from build123d import *

# Parameters (mm, degrees)
BASE_FLANGE1_DEPTH      = 4.4
CUT_EXTRUDE1_DEPTH      = 10.36
CUT_EXTRUDE1_DEPTH_BACK = 4.76
CUT_EXTRUDE2_DEPTH      = 4.76
BOSS_EXTRUDE1_START     = 0.36
BOSS_EXTRUDE1_DEPTH     = 0.36


# Sheet-metal steps are written as plain solids
with BuildPart() as part:
    # Sketch2 → Base-Flange1 (new body)
    with BuildSketch(Plane(origin=(0, 0, 0), x_dir=(1, 0, 0), z_dir=(0, 1, 0))):
        with BuildLine():
            Line((-33.306696524, 16.994496658), (30.293303476, 16.994496658))
            ThreePointArc((30.293303476, 16.994496658), (32.556045176, 16.057238357), (33.493303476, 13.794496658))
            Line((33.493303476, 13.794496658), (33.493303476, -9.805503342))
            ThreePointArc((33.493303476, -9.805503342), (32.556045176, -12.068245042), (30.293303476, -13.005503342))
            Line((30.293303476, -13.005503342), (-33.306696524, -13.005503342))
            ThreePointArc((-33.306696524, -13.005503342), (-35.569438223, -12.068245042), (-36.506696524, -9.805503342))
            Line((-36.506696524, -9.805503342), (-36.506696524, 13.794496658))
            ThreePointArc((-36.506696524, 13.794496658), (-35.569438223, 16.057238357), (-33.306696524, 16.994496658))
        make_face()
    extrude(amount=-BASE_FLANGE1_DEPTH)

    # Sketch7 → Cut-Extrude1 (cut, two sides: drawn at the far end of the back side and taken through both)
    with BuildSketch(Plane(origin=(0, 0, 0), x_dir=(1, 0, 0), z_dir=(0, 1, 0)).offset(-CUT_EXTRUDE1_DEPTH_BACK)):
        with BuildLine():
            Line((-28.006696524, 4.494496658), (-19.506696524, 4.494496658))
            ThreePointArc((-19.506696524, 4.494496658), (-17.006696524, 1.994496658), (-19.506696524, -0.505503342))
            Line((-19.506696524, -0.505503342), (-28.006696524, -0.505503342))
            ThreePointArc((-28.006696524, -0.505503342), (-30.506696524, 1.994496658), (-28.006696524, 4.494496658))
        make_face()
        with BuildLine():
            Line((23.493303476, 4.494496658), (33.493303476, 4.494496658))
            ThreePointArc((33.493303476, 4.494496658), (35.993303476, 1.994496658), (33.493303476, -0.505503342))
            Line((33.493303476, -0.505503342), (23.493303476, -0.505503342))
            ThreePointArc((23.493303476, -0.505503342), (20.993303476, 1.994496658), (23.493303476, 4.494496658))
        make_face()
    extrude(amount=CUT_EXTRUDE1_DEPTH + CUT_EXTRUDE1_DEPTH_BACK, mode=Mode.SUBTRACT)

    # Sketch8 → Cut-Extrude2 (cut)
    with BuildSketch(Plane(origin=(0, 0, 0), x_dir=(1, 0, 0), z_dir=(0, 1, 0))):
        with BuildLine():
            Line((8.293303476, 2.994496658), (8.293303476, -13.005503342))
            ThreePointArc((8.293303476, -13.005503342), (1.993303476, -19.305503342), (-4.306696524, -13.005503342))
            Line((-4.306696524, -13.005503342), (-4.306696524, 2.994496658))
            ThreePointArc((-4.306696524, 2.994496658), (1.993303476, 9.294496658), (8.293303476, 2.994496658))
        make_face()
    extrude(amount=-CUT_EXTRUDE2_DEPTH, mode=Mode.SUBTRACT)

    # Sketch11 → Boss-Extrude1 (add)
    with BuildSketch(Plane(origin=(0, 0, 0), x_dir=(1, 0, 0), z_dir=(0, 1, 0)).offset(BOSS_EXTRUDE1_START)):
        with BuildLine():
            Line((-36.506696524, 13.794496658), (-36.506696524, -9.805503342))
            ThreePointArc((-36.506696524, -9.805503342), (-35.569438223, -12.068245042), (-33.306696524, -13.005503342))
            Line((-33.306696524, -13.005503342), (-7.006696524, -13.005503342))
            Line((-7.006696524, -13.005503342), (-7.006696524, 2.994496658))
            ThreePointArc((-7.006696524, 2.994496658), (1.993303476, 11.994496658), (10.993303476, 2.994496658))
            Line((10.993303476, 2.994496658), (10.993303476, -13.005503342))
            Line((10.993303476, -13.005503342), (30.293303476, -13.005503342))
            ThreePointArc((30.293303476, -13.005503342), (32.556045176, -12.068245042), (33.493303476, -9.805503342))
            Line((33.493303476, -9.805503342), (33.493303476, -0.505503342))
            Line((33.493303476, -0.505503342), (23.493303476, -0.505503342))
            ThreePointArc((23.493303476, -0.505503342), (20.993303476, 1.994496658), (23.493303476, 4.494496658))
            Line((23.493303476, 4.494496658), (33.493303476, 4.494496658))
            Line((33.493303476, 4.494496658), (33.493303476, 13.794496658))
            ThreePointArc((33.493303476, 13.794496658), (32.556045176, 16.057238357), (30.293303476, 16.994496658))
            Line((30.293303476, 16.994496658), (-33.306696524, 16.994496658))
            ThreePointArc((-33.306696524, 16.994496658), (-35.569438223, 16.057238357), (-36.506696524, 13.794496658))
        make_face()
        with BuildLine():
            Line((-19.506696524, 4.494496658), (-28.006696524, 4.494496658))
            ThreePointArc((-28.006696524, 4.494496658), (-30.506696524, 1.994496658), (-28.006696524, -0.505503342))
            Line((-28.006696524, -0.505503342), (-19.506696524, -0.505503342))
            ThreePointArc((-19.506696524, -0.505503342), (-17.006696524, 1.994496658), (-19.506696524, 4.494496658))
        make_face(mode=Mode.SUBTRACT)
    extrude(amount=-BOSS_EXTRUDE1_DEPTH)


solid = part.part
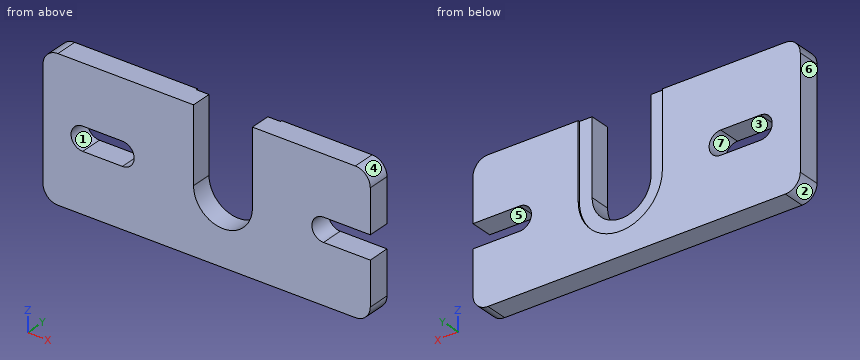
Could you check a few things on this model? Use its own coordinates, in mm. Face numbers are marked on the shaded views. A direction names the side the tool comes from. Give positions to 0.01 mm unless a question says otherwise; leave off trailing zeros. Order: outer loops, then holes, each group sorted by start corner. A loop starts at its lowest first (then second) coordinate and runs counter-clockwise, first axis right, second up. Notation, with made-up numbers: (-30.75, 70) - (20.25, 70) arc R38 cw to (20.25, 109) - close; hole circle Ø9 at (44, -33). An arc over 180 degrees is marked (long way). One line per question, with ' | ' between items. Start each with the question number.
Item 1: I want a section at A-A on z = 6. Write out the boundary of the cut face in (x, y), then the cut area to 3 significant figures.
Item 2: For the marked faces 5, 6 and 7, which set-ups out of +Z, -Z, +X, -X, +Y, -Y let a thin tool reach every point of the face, with its end or its side?
Item 3: I want a section at D-D on z = -1. Write out the boundary of the cut face in (x, y), then the cut area to 3 significant figures.
Item 4: I want a section at B-B on x = -21. Write out the boundary of the cut face in (y, z), then the cut area to 3 significant figures.
Item 5: I'm going to push flat-ended pins straight in: pin 1 Ø1 at (x, z) = (9.5, -1.5) entering from +Y; pin 2 Ø1.5 at (x, z) = (-0.5, -6) entering from +Y. Where does each tip first touch, or does it pass through?
Item 6: I need wall thicknesses on probe 1 along X at (y, z) = (-3.65, 7); probe 2 along Z at (x, y) = (24.5, -2.4); probe 3 along X at (y, z) = (-1.45, -2.75). Which ranges of each line are inside material? Lowest first, please. Write a range as [from, to].
Item 7: Thinking about a two-plate mould opening in X: for the marked faces 1, 2, 3 and 4, which applies, pulls with the +X half, pulls with the -X half, needs draft (parallel to the pull), parting line crosses it, or undercut?
Item 8: I want a section at C-C on y = -1.4. Write out the boundary of the cut face in (x, z).
Verdict:
1) outline: (-36.51, -4.4) - (-4.31, -4.4) - (-4.31, 0) - (-7.01, 0) - (-7.01, 0.36) - (-36.51, 0.36) - close; (8.29, -4.4) - (33.49, -4.4) - (33.49, 0.36) - (10.99, 0.36) - (10.99, 0) - (8.29, 0) - close | area: 271 mm^2
2) face 5: +X, +Y, -Y | face 6: +Z, -Z, -X, +Y, -Y | face 7: +Y, -Y
3) outline: (-36.51, -4.4) - (-30.3, -4.4) - (-30.3, 0.36) - (-36.51, 0.36) - close; (-17.21, -4.4) - (-4.31, -4.4) - (-4.31, 0) - (-7.01, 0) - (-7.01, 0.36) - (-17.21, 0.36) - close; (8.29, -4.4) - (21.2, -4.4) - (21.2, 0.36) - (10.99, 0.36) - (10.99, 0) - (8.29, 0) - close | area: 150 mm^2
4) outline: (-4.4, -16.99) - (0.36, -16.99) - (0.36, -4.49) - (-4.4, -4.49) - close; (-4.4, 0.51) - (0.36, 0.51) - (0.36, 13.01) - (-4.4, 13.01) - close | area: 119 mm^2
5) pin 1: y = 0 | pin 2: through
6) probe 1: [-36.51, -4.31], [8.29, 33.49] | probe 2: [-16.99, -4.49], [0.51, 13.01] | probe 3: [-36.51, -30.39], [-17.12, -4.31], [8.29, 21.11]
7) face 1: undercut | face 2: pulls with the -X half | face 3: undercut | face 4: pulls with the +X half
8) outline: (-36.51, -13.79) arc R3.2 ccw to (-33.31, -16.99) - (30.29, -16.99) arc R3.2 ccw to (33.49, -13.79) - (33.49, -4.49) - (23.49, -4.49) arc R2.5 cw to (23.49, 0.51) - (33.49, 0.51) - (33.49, 9.81) arc R3.2 ccw to (30.29, 13.01) - (8.29, 13.01) - (8.29, -2.99) arc R6.3 cw to (-4.31, -2.99) - (-4.31, 13.01) - (-33.31, 13.01) arc R3.2 ccw to (-36.51, 9.81) - close; hole (-28.01, -4.49) - (-19.51, -4.49) arc R2.5 ccw to (-19.51, 0.51) - (-28.01, 0.51) arc R2.5 ccw to start
